from build123d import *

# Parameters (mm, degrees)
BOSS_EXTRUDE1_DEPTH   = 2
SKETCH1_4_R           = 1.5
BOSS_EXTRUDE2_DEPTH   = 19
BOSS_EXTRUDE2_2_DEPTH = 19
BOSS_EXTRUDE2_3_DEPTH = 19
BOSS_EXTRUDE2_4_DEPTH = 19
BOSS_EXTRUDE2_5_DEPTH = 19
BOSS_EXTRUDE2_6_DEPTH = 19
SKETCH1_5_R           = 1.5
BOSS_EXTRUDE3_DEPTH   = 20
BOSS_EXTRUDE4_DEPTH   = 22
SKETCH2_W             = 23
SKETCH2_H             = 8
SKETCH2_W_2           = 13.5
SKETCH2_H_2           = 13.3
CUT_EXTRUDE1_DEPTH    = 3
SKETCH3_W             = 20
SKETCH3_H             = 12
SKETCH3_W_2           = 33
CUT_EXTRUDE2_DEPTH    = 3
SKETCH4_W             = 12
SKETCH4_H             = 7.5
CUT_EXTRUDE3_DEPTH    = 3
SKETCH10_W            = 190
SKETCH10_H            = 63
SKETCH10_W_2          = 186
SKETCH10_H_2          = 59
BOSS_EXTRUDE5_DEPTH   = 2
SKETCH10_3_W          = 186
SKETCH10_3_H          = 59
CUT_EXTRUDE7_DEPTH    = 22
CUT_EXTRUDE8_DEPTH    = 2
CUT_EXTRUDE9_DEPTH    = 2
CUT_EXTRUDE10_DEPTH   = 2
SKETCH9_W             = 190
SKETCH9_H             = 22
CUT_EXTRUDE11_DEPTH   = 2
SKETCH1_7_R           = 1.5
CUT_EXTRUDE12_DEPTH   = 24


with BuildPart() as part:
    # Sketch1 → Boss-Extrude1 (new body)
    with BuildSketch(Plane(origin=(0, 0, 0), x_dir=(1, 0, 0), z_dir=(0, 1, 0))):
        with BuildLine():
            ThreePointArc((86, 27), (87.318019485, 23.818019485), (90.5, 22.5))
            Line((90.5, 22.5), (93, 22.5))
            Line((93, 22.5), (93, -22.5))
            Line((93, -22.5), (90.5, -22.5))
            ThreePointArc((90.5, -22.5), (87.318019485, -23.818019485), (86, -27))
            Line((86, -27), (86, -29.5))
            Line((86, -29.5), (4.5, -29.5))
            Line((4.5, -29.5), (4.5, -27))
            ThreePointArc((4.5, -27), (0, -22.5), (-4.5, -27))
            Line((-4.5, -27), (-4.5, -29.5))
            Line((-4.5, -29.5), (-86, -29.5))
            Line((-86, -29.5), (-86, -27))
            ThreePointArc((-86, -27), (-87.318019485, -23.818019485), (-90.5, -22.5))
            Line((-90.5, -22.5), (-93, -22.5))
            Line((-93, -22.5), (-93, 22.5))
            Line((-93, 22.5), (-90.5, 22.5))
            ThreePointArc((-90.5, 22.5), (-87.318019485, 23.818019485), (-86, 27))
            Line((-86, 27), (-86, 29.5))
            Line((-86, 29.5), (-4.5, 29.5))
            Line((-4.5, 29.5), (-4.5, 27))
            ThreePointArc((-4.5, 27), (0, 22.5), (4.5, 27))
            Line((4.5, 27), (4.5, 29.5))
            Line((4.5, 29.5), (86, 29.5))
            Line((86, 29.5), (86, 27))
        make_face()
    extrude(amount=BOSS_EXTRUDE1_DEPTH)



with BuildPart() as body_2:
    # Sketch1_4 → Boss-Extrude2 (new body)
    with BuildSketch(Plane(origin=(0, 0, 0), x_dir=(1, 0, 0), z_dir=(0, 1, 0))):
        with Locations(Location((90.5, 27, 0), (0, 0, 270))):
            Circle(SKETCH1_4_R)
    extrude(amount=BOSS_EXTRUDE2_DEPTH)



with BuildPart() as body_3:
    # Sketch1_4 → Boss-Extrude2 2 (new body)
    with BuildSketch(Plane(origin=(0, 0, 0), x_dir=(1, 0, 0), z_dir=(0, 1, 0))):
        with Locations(Location((90.5, -27, 0), (0, 0, 270))):
            Circle(SKETCH1_4_R)
    extrude(amount=BOSS_EXTRUDE2_2_DEPTH)


with BuildPart() as body_4:
    # Sketch1_4 → Boss-Extrude2 3 (new body)
    with BuildSketch(Plane(origin=(0, 0, 0), x_dir=(1, 0, 0), z_dir=(0, 1, 0))):
        with Locations(Location((0, -27, 0), (0, 0, 270))):
            Circle(SKETCH1_4_R)
    extrude(amount=BOSS_EXTRUDE2_3_DEPTH)


with BuildPart() as body_5:
    # Sketch1_4 → Boss-Extrude2 4 (new body)
    with BuildSketch(Plane(origin=(0, 0, 0), x_dir=(1, 0, 0), z_dir=(0, 1, 0))):
        with Locations(Location((0, 27, 0), (0, 0, 270))):
            Circle(SKETCH1_4_R)
    extrude(amount=BOSS_EXTRUDE2_4_DEPTH)


with BuildPart() as body_6:
    # Sketch1_4 → Boss-Extrude2 5 (new body)
    with BuildSketch(Plane(origin=(0, 0, 0), x_dir=(1, 0, 0), z_dir=(0, 1, 0))):
        with Locations(Location((-90.5, 27, 0), (0, 0, 270))):
            Circle(SKETCH1_4_R)
    extrude(amount=BOSS_EXTRUDE2_5_DEPTH)


with BuildPart() as body_7:
    # Sketch1_4 → Boss-Extrude2 6 (new body)
    with BuildSketch(Plane(origin=(0, 0, 0), x_dir=(1, 0, 0), z_dir=(0, 1, 0))):
        with Locations(Location((-90.5, -27, 0), (0, 0, 90))):
            Circle(SKETCH1_4_R)
    extrude(amount=BOSS_EXTRUDE2_6_DEPTH)


with BuildPart() as body_2_1:
    add(body_2.part)

    add(body_3.part)  # Boss-Extrude3 merges body 3

    add(body_4.part)  # Boss-Extrude3 merges body 4

    add(body_5.part)  # Boss-Extrude3 merges body 5

    add(body_6.part)  # Boss-Extrude3 merges body 6

    add(body_7.part)  # Boss-Extrude3 merges body 7
    # Sketch1_5 → Boss-Extrude3 (add)
    with BuildSketch(Plane(origin=(0, 0, 0), x_dir=(1, 0, 0), z_dir=(0, 1, 0))):
        Polygon((93.5, 27), (92, 24.401923789), (89, 24.401923789), (87.5, 27), (89, 29.598076211), (92, 29.598076211), align=None)
        with Locations(Location((90.5, 27, 0), (0, 0, 270))):
            Circle(SKETCH1_5_R, mode=Mode.SUBTRACT)
        Polygon((89, -29.598076211), (92, -29.598076211), (93.5, -27), (92, -24.401923789), (89, -24.401923789), (87.5, -27), align=None)
        with Locations(Location((90.5, -27, 0), (0, 0, 270))):
            Circle(SKETCH1_5_R, mode=Mode.SUBTRACT)
        Polygon((3, -27), (1.5, -29.598076211), (-1.5, -29.598076211), (-3, -27), (-1.5, -24.401923789), (1.5, -24.401923789), align=None)
        with Locations(Location((0, -27, 0), (0, 0, 270))):
            Circle(SKETCH1_5_R, mode=Mode.SUBTRACT)
        Polygon((-1.5, 24.401923789), (1.5, 24.401923789), (3, 27), (1.5, 29.598076211), (-1.5, 29.598076211), (-3, 27), align=None)
        with Locations(Location((0, 27, 0), (0, 0, 270))):
            Circle(SKETCH1_5_R, mode=Mode.SUBTRACT)
        Polygon((-93.5, -27), (-92, -24.401923789), (-89, -24.401923789), (-87.5, -27), (-89, -29.598076211), (-92, -29.598076211), align=None)
        with Locations(Location((-90.5, -27, 0), (0, 0, 90))):
            Circle(SKETCH1_5_R, mode=Mode.SUBTRACT)
        Polygon((-89, 29.598076211), (-92, 29.598076211), (-93.5, 27), (-92, 24.401923789), (-89, 24.401923789), (-87.5, 27), align=None)
        with Locations(Location((-90.5, 27, 0), (0, 0, 270))):
            Circle(SKETCH1_5_R, mode=Mode.SUBTRACT)
    extrude(amount=BOSS_EXTRUDE3_DEPTH)


with BuildPart() as part_1:
    add(part.part)

    add(body_2_1.part)  # Boss-Extrude4 merges body 2
    # Sketch1_6 → Boss-Extrude4 (add)
    with BuildSketch(Plane(origin=(0, 0, 0), x_dir=(1, 0, 0), z_dir=(0, 1, 0))):
        Polygon((-95, -22.5), (-95, -31.5), (-86, -31.5), (86, -31.5), (95, -31.5), (95, -22.5), (95, 22.5), (95, 31.5), (86, 31.5), (4.5, 31.5), (-4.5, 31.5), (-86, 31.5), (-95, 31.5), (-95, 22.5), align=None)
        Polygon((-89, -29.598076211), (-92, -29.598076211), (-93.5, -27), (-92, -24.401923789), (-89, -24.401923789), (-87.5, -27), align=None, mode=Mode.SUBTRACT)
        Polygon((-1.5, -24.401923789), (1.5, -24.401923789), (3, -27), (1.5, -29.598076211), (-1.5, -29.598076211), (-3, -27), align=None, mode=Mode.SUBTRACT)
        Polygon((92, -29.598076211), (89, -29.598076211), (87.5, -27), (89, -24.401923789), (92, -24.401923789), (93.5, -27), align=None, mode=Mode.SUBTRACT)
        Polygon((-92, 24.401923789), (-93.5, 27), (-92, 29.598076211), (-89, 29.598076211), (-87.5, 27), (-89, 24.401923789), align=None, mode=Mode.SUBTRACT)
        Polygon((1.5, 29.598076211), (3, 27), (1.5, 24.401923789), (-1.5, 24.401923789), (-3, 27), (-1.5, 29.598076211), align=None, mode=Mode.SUBTRACT)
        with BuildLine():
            Line((-93, -22.5), (-93, 22.5))
            Line((-93, 22.5), (-90.5, 22.5))
            ThreePointArc((-90.5, 22.5), (-87.318019485, 23.818019485), (-86, 27))
            Line((-86, 27), (-86, 29.5))
            Line((-86, 29.5), (-4.5, 29.5))
            Line((-4.5, 29.5), (-4.5, 27))
            ThreePointArc((-4.5, 27), (0, 22.5), (4.5, 27))
            Line((4.5, 27), (4.5, 29.5))
            Line((4.5, 29.5), (86, 29.5))
            Line((86, 29.5), (86, 27))
            ThreePointArc((86, 27), (87.318019485, 23.818019485), (90.5, 22.5))
            Line((90.5, 22.5), (93, 22.5))
            Line((93, 22.5), (93, -22.5))
            Line((93, -22.5), (90.5, -22.5))
            ThreePointArc((90.5, -22.5), (87.318019485, -23.818019485), (86, -27))
            Line((86, -27), (86, -29.5))
            Line((86, -29.5), (4.5, -29.5))
            Line((4.5, -29.5), (4.5, -27))
            ThreePointArc((4.5, -27), (0, -22.5), (-4.5, -27))
            Line((-4.5, -27), (-4.5, -29.5))
            Line((-4.5, -29.5), (-86, -29.5))
            Line((-86, -29.5), (-86, -27))
            ThreePointArc((-86, -27), (-87.318019485, -23.818019485), (-90.5, -22.5))
            Line((-90.5, -22.5), (-93, -22.5))
        make_face(mode=Mode.SUBTRACT)
        Polygon((89, 29.598076211), (92, 29.598076211), (93.5, 27), (92, 24.401923789), (89, 24.401923789), (87.5, 27), align=None, mode=Mode.SUBTRACT)
    extrude(amount=BOSS_EXTRUDE4_DEPTH)

    # Sketch2 → Cut-Extrude1 (cut)
    with BuildSketch(Plane(origin=(95, 0, 0), x_dir=(0, 0, -1), z_dir=(1, 0, 0))):
        with Locations((-10, 6)):
            Rectangle(SKETCH2_W, SKETCH2_H)
        with Locations((14.75, 8.65)):
            Rectangle(SKETCH2_W_2, SKETCH2_H_2)
    extrude(amount=-CUT_EXTRUDE1_DEPTH, mode=Mode.SUBTRACT)

    # Sketch3 → Cut-Extrude2 (cut)
    with BuildSketch(Plane(origin=(0, 0, -31.5), x_dir=(-1, 0, 0), z_dir=(0, 0, -1))):
        with Locations((-65, 8)):
            Rectangle(SKETCH3_W, SKETCH3_H)
        with Locations((51.5, 8)):
            Rectangle(SKETCH3_W_2, SKETCH3_H)
    extrude(amount=-CUT_EXTRUDE2_DEPTH, mode=Mode.SUBTRACT)

    # Sketch4 → Cut-Extrude3 (cut)
    with BuildSketch(Plane.ZY.offset(95)):
        with Locations((-9.5, 5.75)):
            Rectangle(SKETCH4_W, SKETCH4_H)
        with Locations((9.5, 5.75)):
            Rectangle(SKETCH4_W, SKETCH4_H)
    extrude(amount=-CUT_EXTRUDE3_DEPTH, mode=Mode.SUBTRACT)

    # Sketch10 → Boss-Extrude5 (add)
    with BuildSketch(Plane(origin=(0, 22, 0), x_dir=(1, 0, 0), z_dir=(0, 1, 0))):
        Rectangle(SKETCH10_W, SKETCH10_H)
        Rectangle(SKETCH10_W_2, SKETCH10_H_2, mode=Mode.SUBTRACT)
        Rectangle(SKETCH10_W_2, SKETCH10_H_2)
    extrude(amount=BOSS_EXTRUDE5_DEPTH)

    # Sketch10_3 → Cut-Extrude7 (cut)
    with BuildSketch(Plane(origin=(0, 22, 0), x_dir=(1, 0, 0), z_dir=(0, 1, 0))):
        Rectangle(SKETCH10_3_W, SKETCH10_3_H)
    extrude(amount=-CUT_EXTRUDE7_DEPTH, mode=Mode.SUBTRACT)

    # Sketch5 → Cut-Extrude8 (cut)
    with BuildSketch(Plane(origin=(95, 0, 0), x_dir=(0, 0, -1), z_dir=(1, 0, 0))):
        Polygon((-21.5, 10), (-21.5, 22), (-31.5, 22), (-31.5, 0), (31.5, 0), (31.5, 22), (21.5, 22), (21.5, 15.3), (8, 15.3), (8, 10), align=None)
    extrude(amount=-CUT_EXTRUDE8_DEPTH, mode=Mode.SUBTRACT)

    # Sketch6 → Cut-Extrude9 (cut)
    with BuildSketch(Plane(origin=(0, 0, -31.5), x_dir=(-1, 0, 0), z_dir=(0, 0, -1))):
        Polygon((-75, 22), (-75, 14), (-55, 14), (-55, 22), (35, 22), (35, 14), (68, 14), (68, 22), (95, 22), (95, 0), (-95, 0), (-95, 22), align=None)
    extrude(amount=-CUT_EXTRUDE9_DEPTH, mode=Mode.SUBTRACT)

    # Sketch7 → Cut-Extrude10 (cut)
    with BuildSketch(Plane.ZY.offset(95)):
        Polygon((-15.5, 9.5), (-15.5, 22), (-31.5, 22), (-31.5, 0), (31.5, 0), (31.5, 22), (15.5, 22), (15.5, 9.5), align=None)
    extrude(amount=-CUT_EXTRUDE10_DEPTH, mode=Mode.SUBTRACT)

    # Sketch9 → Cut-Extrude11 (cut)
    with BuildSketch(Plane.XY.offset(31.5)):
        with Locations((0, 11)):
            Rectangle(SKETCH9_W, SKETCH9_H)
    extrude(amount=-CUT_EXTRUDE11_DEPTH, mode=Mode.SUBTRACT)

    # Sketch1_7 → Cut-Extrude12 (cut)
    with BuildSketch(Plane(origin=(0, 0, 0), x_dir=(1, 0, 0), z_dir=(0, 1, 0))):
        with Locations(Location((-90.5, -27, 0), (0, 0, 270))):
            Circle(SKETCH1_7_R)
        with Locations(Location((-90.5, 27, 0), (0, 0, 270))):
            Circle(SKETCH1_7_R)
        with Locations(Location((90.5, -27, 0), (0, 0, 270))):
            Circle(SKETCH1_7_R)
        with Locations(Location((90.5, 27, 0), (0, 0, 270))):
            Circle(SKETCH1_7_R)
        with Locations(Location((0, -27, 0), (0, 0, 270))):
            Circle(SKETCH1_7_R)
        with Locations(Location((0, 27, 0), (0, 0, 270))):
            Circle(SKETCH1_7_R)
    extrude(amount=CUT_EXTRUDE12_DEPTH, mode=Mode.SUBTRACT)


solid = part_1.part
Could you check a few things on this model? Use its own coordinates, in mm. A direction names the side the tool comes from. Round coordinates to 2 decimals unless told otherwise and drop trailing zeros. Order: outer loops, then holes, each group sorted by start corner. A loop starts at its lowest first (then second) coordinate and runs counter-clockwise, first axis right, second up.
(1) Imagine slicing it at C-C (x = -63). Write out the boundary of the cut face in (y, z).
Response values:
outline: (14, -31.5) - (24, -31.5) - (24, 31.5) - (22, 31.5) - (22, -29.5) - (14, -29.5) - close
(2) I'm going to push flat-ended pins straight in: pin 1 (1.6 mm diameter, centred on y = 18.5, z = -31, fed in from -X); pin 2 (2.5 mm diameter, centred on x = -47, y = 18.5, fed in from +Z); pin 3 (2 mm diameter, centred on x = 94, z = 7.5, fed in from -Y); pin 4 (3.5 mm diameter, centred on x = -90.5, z = 27, fed in from +Y). Where does each tip first touch, or does it pass through?
Response values:
pin 1: stops at x = -68
pin 2: stops at z = -29.5
pin 3: stops at y = 10
pin 4: stops at y = 24
(3) Please list where these lines run through material, in increasing order: line 1 along X through (y, z) = (22.5, -27); line 2 along Z through (x, y) = (-90.5, 22.9); line 3 along X through (y, z) = (21.75, 3.5).
Response values:
line 1: x = -95 to -92, -89 to -1.5, 1.5 to 89, 92 to 95
line 2: z = -31.5 to -28.5, -25.5 to 25.5, 28.5 to 31.5
line 3: x = -95 to -93, 93 to 95
(4) Imagine slicing it at B-B (z = 0). Write out the boundary of the cut face in (x, y).
Response values:
outline: (-95, 9.5) - (-93, 9.5) - (-93, 22) - (93, 22) - (93, 10) - (95, 10) - (95, 24) - (-95, 24) - close
(5) Imagine slicing it at A-A (y = 12). Write out the boundary of the cut face in (x, z).
Response values:
outline: (-95, -15.5) - (-93, -15.5) - (-93, 15.5) - (-95, 15.5) - close; (93, -8) - (95, -8) - (95, 21.5) - (93, 21.5) - close
(6) If we mould it in two halves opening along X, with no side actions, what happens to faces 4 (the flat face through (-95, 17, 0)), 5 (the flat face through (-1, 24, 0)), 6 (the flat face through (-1, 22, 0))? For each: released by +X, released by -X, zero draft, split by the parting line, or undercut.
Response values:
face 4: released by -X
face 5: zero draft
face 6: undercut
(7) Which directions (+Z, -Z, +X, -X, +Y, -Y) give clear straight access to the entire face, cutting with the end or side of a thin tool? Please do faces 1 (the flat face through (95, 17, 0)), 2 (the flat face through (-93, 16, 0)), 3 (the flat face through (65, 18, -29.5)).
Response values:
face 1: +Z, -Z, +X, +Y, -Y
face 2: +Z, -Z, -Y
face 3: +Z, +X, -X, -Y
